Verification items for this drawing (mm, ordinates from the low corner). A direction names the side the tool comes from. Round coordinates to 2 decimals unless told otherwise and drop trailing zeros. Loops run counter-clockwise (first coordinate to the right, second up) from the corner with the lowest first, then second, coordinate; pieces in that order, holes last. Notation, with made-up numbers: M 21.5,75.5 L 29.5,75.5 A10 ccw 29.5,90.5 Z; hole C 63,-40 d9. An arc over 180 degrees is marked long. Write item = value, one per line. Start each with the question number.
(1) Cross-section at C-C on y = 4. Record the boundary of the cut face in (x, z).
(2) Cross-section at B-B on z = 15. Record the boundary of the cut face in (x, y).
(3) Cross-section at D-D on x = 3. Record the boundary of the cut face in (y, z).
(4) Scan lines: L1, parallel to X at y = 11.43, z = 0.8 (1 decimal); L2, parallel to X at y = 15.75, z = 30; L3, parallel to Z at x = 17.5, y = 5. Record each from-to range of solid material in increasing order. Write a range as from..to.
(5) Set-up check for the marked faces 1 and 2: record each of +Z, -Z, +X, -X, +Y, -Y from which the full face is reachable in a straight line by a thin tool's end or side.
(6) Cross-section at A-A on x = 10.16. Record the boundary of the cut face in (y, z) (1 decimal).
(7) Go/stop test with flat-tipped pins: P1, Ø11.5, axis at x = 23, y = 11, coming from the +Z side; P2, Ø10, axis at y = 16.5, z = 10, coming from the -X side. Record where each tip stops, or that it passes through.
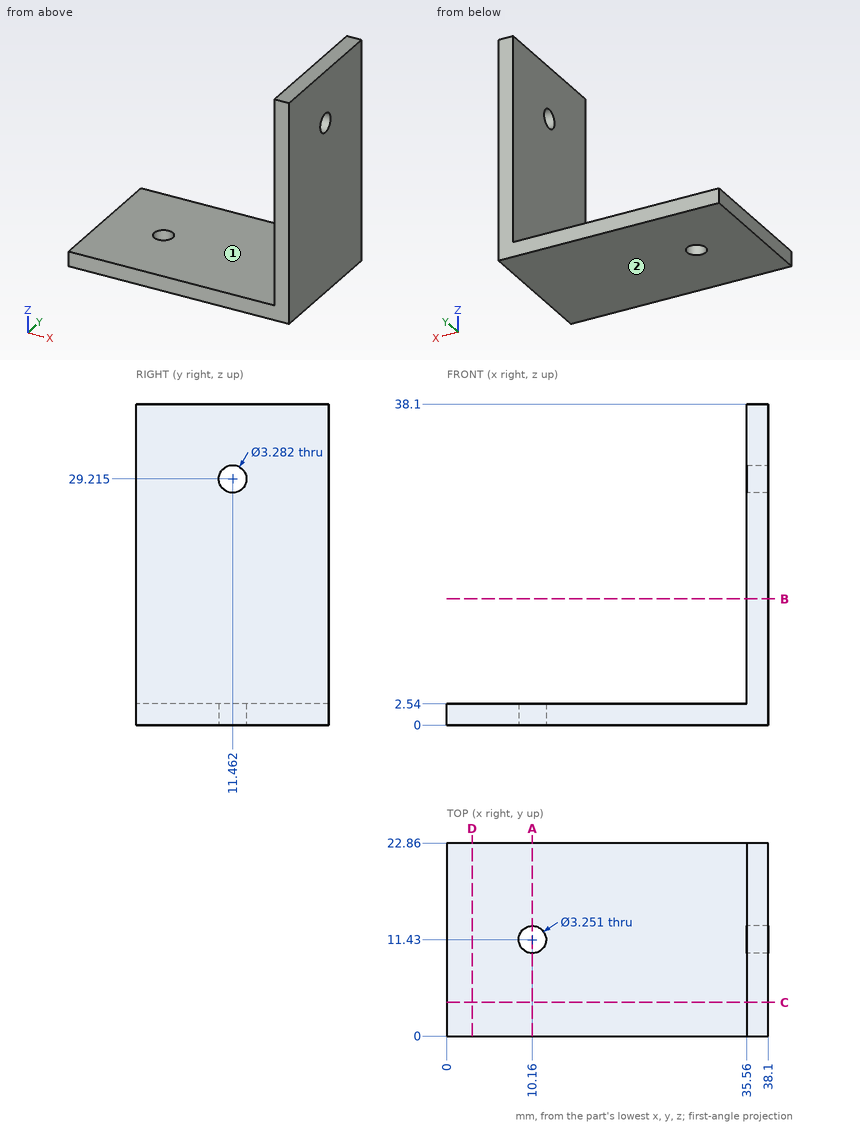
Result:
q1.outline = M 0,0 L 38.1,0 L 38.1,38.1 L 35.56,38.1 L 35.56,2.54 L 0,2.54 Z
q2.outline = M 35.56,0 L 38.1,0 L 38.1,22.86 L 35.56,22.86 Z
q3.outline = M 0,0 L 22.86,0 L 22.86,2.54 L 0,2.54 Z
q4.L1 = 0..8.5, 11.8..38.1
q4.L2 = 35.56..38.1
q4.L3 = 0..2.54
q5.face_1 = +Z, -X, +Y, -Y
q5.face_2 = -Z, +X, -X, +Y, -Y
q6.outline = M 0,0 L 9.8,0 L 9.8,2.5 L 0,2.5 Z; M 13.1,0 L 22.9,0 L 22.9,2.5 L 13.1,2.5 Z
q7.P1 = 2.54
q7.P2 = 35.56
